The listing builds one solid part. Answer for the finished solid, in the listing's coordinates (mm). Face numbers are marked on the shaded views. A direction names the side the tool comes from. Give positions to 0.01 mm unless a question says otherwise; leave off trailing zeros. Loops run counter-clockwise (first coordinate to the right, second up) from the corner with the lowest first, then second, coordinate; pieces in that order, holes last. Notation, with made-up numbers: (76.5, -6) - (134.5, -6) arc R15 ccw to (134.5, 17) - close; hole circle Ø4 at (-14.75, -18.75). An arc over 180 degrees is marked (long way). Answer in a Markdown table with one row per item. Add a question column.
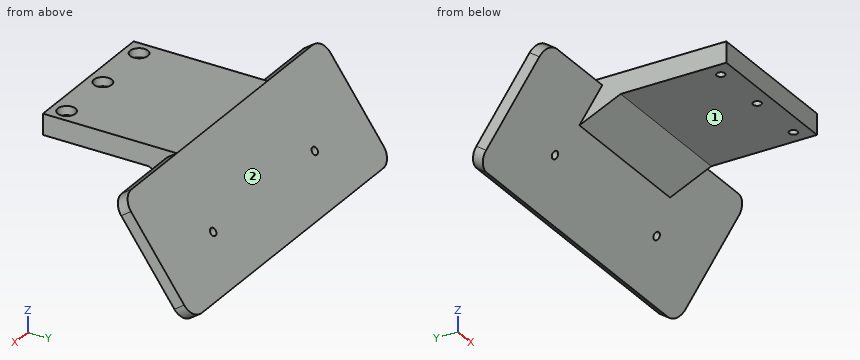
```python
from build123d import *

# Parameters (mm, degrees)
SKETCH_1_W          = 50
SKETCH_1_H          = 7
EXTRUDE_1_DEPTH     = 45
SKETCH_2_R          = 3
CUT_EXTRUDE_1_DEPTH = 3
SKETCH_3_R          = 1.4
CUT_EXTRUDE_2_DEPTH = 83.08499944
SKETCH_5_R          = 1.3
EXTRUDE_2_DEPTH     = 4.015035
EXTRUDE_3_DEPTH     = 50
FILLET_1_R          = 5


with BuildPart() as part:
    # 草图1 → 凸台-拉伸1 (new body)
    with BuildSketch(Plane(origin=(0, 0, 0), x_dir=(1, 0, 0), z_dir=(0, 1, 0))):
        with Locations((-43.534277066, -15.400769649)):
            Rectangle(SKETCH_1_W, SKETCH_1_H)
    extrude(amount=EXTRUDE_1_DEPTH)

    # 草图2 → 切除-拉伸1 (cut)
    with BuildSketch(Plane.XY.offset(18.900769649)):
        with Locations((-43.350176606, 5)):
            Circle(SKETCH_2_R)
        with Locations((-23.350176606, 5)):
            Circle(SKETCH_2_R)
        with Locations((-63.350176606, 5)):
            Circle(SKETCH_2_R)
    extrude(amount=-CUT_EXTRUDE_1_DEPTH, mode=Mode.SUBTRACT)

    # 草图3 → 切除-拉伸2 (cut, through all)
    with BuildSketch(Plane.XY.offset(15.900769649)):
        with Locations((-23.350176606, 5)):
            Circle(SKETCH_3_R)
        with Locations((-43.350176606, 5)):
            Circle(SKETCH_3_R)
        with Locations((-63.350176606, 5)):
            Circle(SKETCH_3_R)
    extrude(amount=-CUT_EXTRUDE_2_DEPTH, mode=Mode.SUBTRACT)

    # 草图5 → 凸台-拉伸2 (add)
    with BuildSketch(Plane(origin=(0, 39.075910108, 27.36124682), x_dir=(1, 0, 0), z_dir=(0, 0.819152044288991, 0.5735764363510473))):
        Polygon((-68.534277066, 10.328335539), (-18.534277066, 10.328335539), (11.465722934, 10.328335539), (11.465722934, 51.520032107), (-18.534277066, 51.520032107), (-68.534277066, 51.520032107), (-98.534277066, 51.520032107), (-98.534277066, 10.328335539), align=None)
        with Locations(Location((-71.375176606, 35.020032107, 0), (0, 0, 270))):
            Circle(SKETCH_5_R, mode=Mode.SUBTRACT)
        with Locations(Location((-15.325176606, 35.020032107, 0), (0, 0, 270))):
            Circle(SKETCH_5_R, mode=Mode.SUBTRACT)
    extrude(amount=-EXTRUDE_2_DEPTH)

    # 草图6 → 凸台-拉伸3 (add)
    with BuildSketch(Plane(origin=(-18.534277066, 0, 0), x_dir=(0, 0, -1), z_dir=(1, 0, 0))):
        Polygon((-11.900769649, 45), (-5.610910777, 49.404206597), (-11.900769649, 35.535742762), align=None)
    extrude(amount=-EXTRUDE_3_DEPTH)

    # 圆角1
    fillet_1_edges = [part.edges().sort_by_distance(p)[0] for p in [
        (11.465722934, 43.355537936, 17.749304916),
        (-98.534277066, 66.982124461, -15.992957536),
        (11.465722934, 66.982124461, -15.992957536),
        (-98.534277066, 43.355537936, 17.749304916),
    ]]
    fillet(fillet_1_edges, radius=FILLET_1_R)


solid = part.part
```
(1) A cutting plane is placed at A-A on y = 5. Determine the outline of the cut face in (x, z), plus the area to 3 significant figures.
(2) A cutting plane is placed at B-B on x = -29. Determine the outline of the cut face in (y, z), plus the area to 3 significant figures.
(3) A tool of negligible diameter and unlimited length cuts with its end or side. For the marked faces 1 and 2, from which of +Z, -Z, +X, -X, +Y, -Y can it reach the whole face along a straight path? Write none if from no direction.
(4) Find the intervals of material crossed by line 1 along Z through (x, y) = (-34, 16); line 2 along X through (y, z) = (43.5, 13); line 3 along Y through (x, z) = (-55, -6), in increasing order. Write a range as [from, to].
(5) Given pin 1 Ø8 at (x, y) = (-46.5, 14) entering from -Z; pin 2 Ø8 at (x, z) = (-30.5, -3) entering from -Y; pin 3 Ø10.5 at (y, z) = (33, 9.5) entering from -X; pin 4 Ø2 at (x, y) = (-63.35, 5) entering from -Z, each flat-ended and moving along its own axis, determine where each tip first touches the part or whether it passes through.
(6) A cutting plane is placed at C-C on y = 30.5. Determine the outline of the cut face in (x, z).
(7) A cutting plane is placed at D-D on z = -9.5. Determine the outline of the cut face in (x, y).
Evaluation:
| question | item | result |
|---|---|---|
| 1 | outline | (-68.53, 11.9) - (-64.75, 11.9) - (-64.75, 15.9) - (-66.35, 15.9) - (-66.35, 18.9) - (-68.53, 18.9) - close; (-61.95, 11.9) - (-44.75, 11.9) - (-44.75, 15.9) - (-46.35, 15.9) - (-46.35, 18.9) - (-60.35, 18.9) - (-60.35, 15.9) - (-61.95, 15.9) - close; (-41.95, 11.9) - (-24.75, 11.9) - (-24.75, 15.9) - (-26.35, 15.9) - (-26.35, 18.9) - (-40.35, 18.9) - (-40.35, 15.9) - (-41.95, 15.9) - close; (-21.95, 11.9) - (-18.53, 11.9) - (-18.53, 18.9) - (-20.35, 18.9) - (-20.35, 15.9) - (-21.95, 15.9) - close |
| 1 | area | 262 mm² |
| 2 | outline | (0, 11.9) - (35.54, 11.9) - (49.4, 5.61) - (65.34, -17.14) - (68.63, -14.84) - (45, 18.9) - (0, 18.9) - close |
| 2 | area | 499 mm² |
| 3 | face 1 | -Z, +X, -X, -Y |
| 3 | face 2 | +Z, +X, -X, +Y |
| 4 | line 1 | z = [11.9, 18.9] |
| 4 | line 2 | x = [-68.53, -18.53] |
| 4 | line 3 | y = [57.53, 62.44] |
| 5 | pin 1 | stops at z = 11.9 |
| 5 | pin 2 | stops at y = 52.63 |
| 5 | pin 3 | stops at x = -68.53 |
| 5 | pin 4 | passes through |
| 6 | outline | (-68.53, 11.9) - (-18.53, 11.9) - (-18.53, 18.9) - (-68.53, 18.9) - close |
| 7 | outline | (-98.53, 59.98) - (11.47, 59.98) - (11.47, 64.89) - (-98.53, 64.89) - close |
